Answer from the drawing. Dimensions are ordinates in mm from the lowest x, y and z of the part. A direction names the side the tool comes from. Coordinates: 2 decimals unless noted, no trailing zeros. Write each loop counter-clockwise with the first axis right and the second up, starting at its lowest first coordinate (ties: lowest second). Pieces come first, ordered by that corner, then holes.
(1) Given pin 1 (1 mm diameter, centred on y = 7, z = 1, fed in from -X); pin 2 (1 mm diameter, centred on y = 2, z = 0.5, fed in from +X), each flat-ended and moving along its own axis, determine where each tip first touches the part or whether it passes through.
(2) Section A-A on x = 2.35 is taken. Write down the section's boundary in (y, z), then the cut area to 3 significant figures.
(3) Which of the six approach directions +Z, -Z, +X, -X, +Y, -Y give full straight-line access (tool end or side, diameter ignored) to the marked faces 1, 2, 3, 4 and 5?
(4) Section C-C on y = 1.25 is taken. Write down the section's boundary in (x, z), then the cut area to 3 significant figures.
(5) Section B-B on y = 8 is taken. Write down the section's boundary in (x, z).
(6) The mould has two halves that part along Y. Classify the marked faces 6, 7 and 8: +Y half, -Y half, draft (parallel to the pull), parting line (faces both ways), or undercut.
(7) Find the intervals of material crossed by probe 1 along Y at (x, z) = (0.9, 0.7); probe 2 along Y at (x, z) = (0.35, 0.65); probe 3 along X at (y, z) = (3, 1.45), in increasing order.
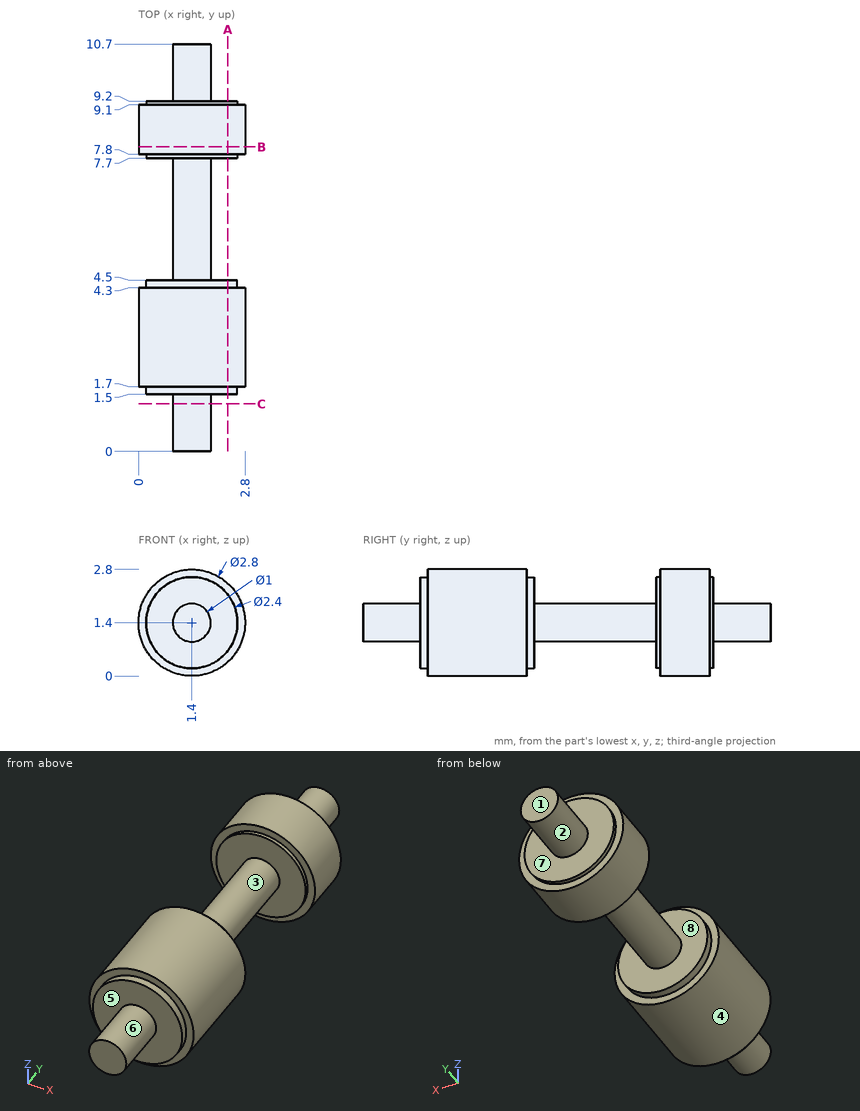
Response:
1. pin 1: stops at x = 0.9
1. pin 2: stops at x = 2.74
2. outline: (1.5, 0.67) - (1.7, 0.67) - (1.7, 0.37) - (4.3, 0.37) - (4.3, 0.67) - (4.5, 0.67) - (4.5, 2.13) - (4.3, 2.13) - (4.3, 2.43) - (1.7, 2.43) - (1.7, 2.13) - (1.5, 2.13) - close; (7.7, 0.67) - (7.8, 0.67) - (7.8, 0.37) - (9.1, 0.37) - (9.1, 0.67) - (9.2, 0.67) - (9.2, 2.13) - (9.1, 2.13) - (9.1, 2.43) - (7.8, 2.43) - (7.8, 2.13) - (7.7, 2.13) - close
2. area: 8.90 mm2
3. face 1: +Z, -Z, +X, -X, +Y
3. face 2: +Y
3. face 3: none
3. face 4: +Y, -Y
3. face 5: -Y
4. outline: circle Ø1 at (1.4, 1.4)
4. area: 0.785 mm2
5. outline: circle Ø2.8 at (1.4, 1.4)
6. face 6: draft
6. face 7: +Y half
6. face 8: undercut
7. probe 1: y = 1.5 to 4.5, 7.7 to 9.2
7. probe 2: y = 1.7 to 4.3, 7.8 to 9.1
7. probe 3: x = 0 to 2.8
